Geometry: see drawing. Coordinates: mm, zero at the bounding-box minimum. Give positions to 0.01 mm unless a question says otherwise; leave off trailing zeros. Write each loop counter-clockwise with the first axis right and the second up, starting at its lowest first coordinate (ties: lowest second). Pieces come first, ordered by that corner, then holes. Notation, with made-up numbers: M 17.5,38 L 26.5,38 A23 ccw 26.5,51 Z; hole C -20,26.25 d3. An arc over 180 degrees is marked long. Use a Markdown table: item, result. Add a question column.
(1) Material intervals for L1, parallel to Y at x = 12.5, z = 1.25 (1 decimal); L2, parallel to Y at x = 16.75, z = 0.65 (1 decimal); L3, parallel to X at y = 26, z = 0.65 (1 decimal), sorted ascending.
(2) Cut plane D-D (y = 13). Output: boundary loops of the cut face in (x, z) (1 decimal).
(3) Cut plane A-A (y = 25.5). Output: boundary loops of the cut face in (x, z).
(4) Cut plane B-B (x = 21.5). Output: boundary loops of the cut face in (y, z) (1 decimal), plus the area to 3 significant figures.
(5) Cut plane C-C (z = 1.2). State how many separate pieces and enclosed holes the cut face has, plus the area to 3 significant figures.
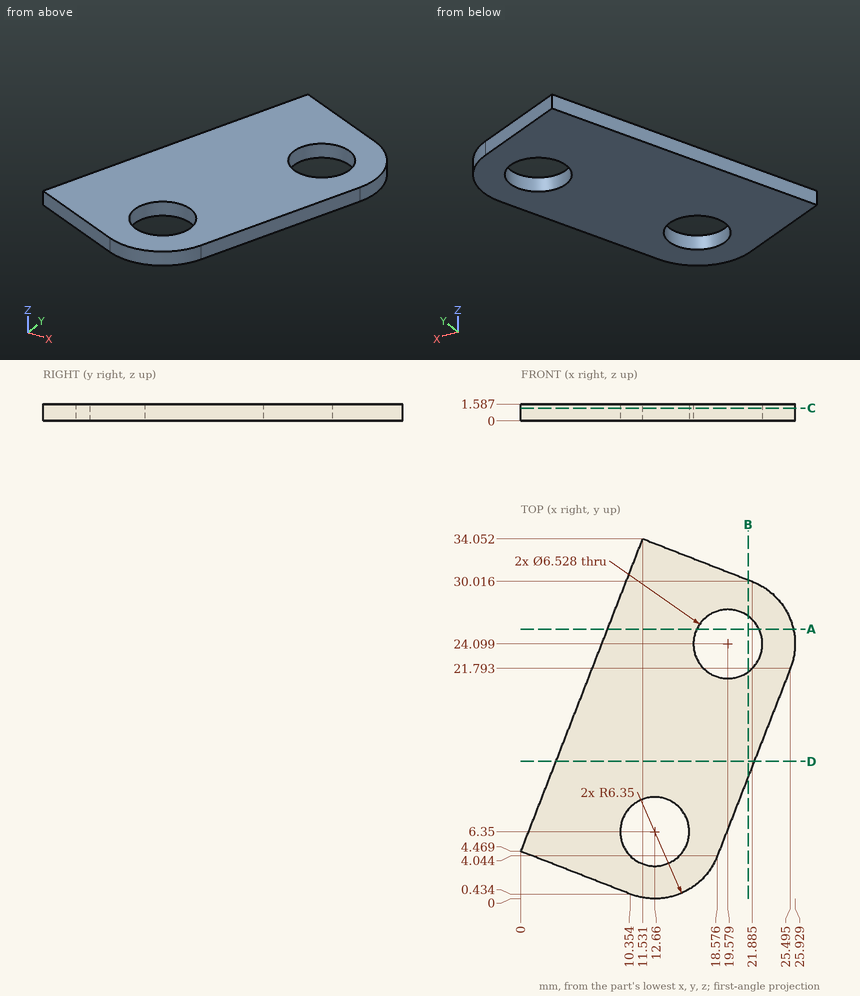
Answer list:
| question | item | result |
|---|---|---|
| 1 | L1 | 0 to 3.1, 9.6 to 33.7 |
| 1 | L2 | 1.5 to 22.5, 25.7 to 32 |
| 1 | L3 | 8.4 to 16.9, 22.2 to 25.6 |
| 2 | outline | M 3.3,0 L 22.1,0 L 22.1,1.6 L 3.3,1.6 Z |
| 3 | outline | M 8.2,0 L 16.63,0 L 16.63,1.59 L 8.2,1.59 Z; M 22.53,0 L 25.77,0 L 25.77,1.59 L 22.53,1.59 Z |
| 4 | outline | M 11.5,0 L 21.5,0 L 21.5,1.6 L 11.5,1.6 Z; M 26.7,0 L 30.2,0 L 30.2,1.6 L 26.7,1.6 Z |
| 4 | area | 21.2 mm² |
| 5 | separate pieces | 1 |
| 5 | enclosed holes | 2 |
| 5 | area | 470 mm² |
